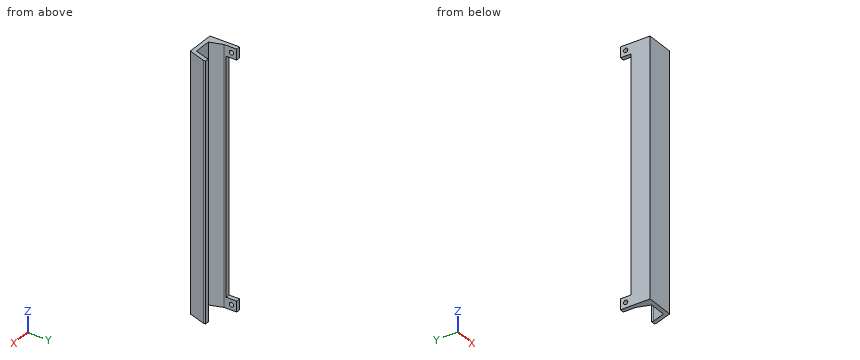
Autodesk Inventor part; units mm, degrees
ref_plane "YZ Plane" through (0, 0, 0) normal (1, 0, 0) x (0, 1, 0)
ref_plane "XZ Plane" through (0, 0, 0) normal (0, 1, 0) x (-1, 0, 0)
ref_plane "XY Plane" through (0, 0, 0) normal (0, 0, 1) x (1, 0, 0)
sketch "Sketch1" plane through (0, 0, 0) normal (0, 0, 1) x (1, 0, 0)
  circle A0 centre (0, 0) radius 7.62
  line L0 (-7.62, 0) -> (-7.62, 1.27)
  line L1 (0, -7.62) -> (-5.08, -7.62)
  line L2 (0, -7.62) -> (5.08, -7.62)
  line L3 (-7.62, 0) -> (-5.08, -7.62)
  line L4 (5.08, -7.62) -> (7.62, 0)
  line L5 (7.62, 0) -> (7.62, 1.27)
  line L6 (-7.62, 1.27) -> (-10.16, 1.27)
  line L7 (-10.16, 1.27) -> (-10.16, 0)
  line L8 (-5.08, -7.62) -> (-6.7733, -10.16)
  line L9 (-6.7733, -10.16) -> (-10.16, 0)
  line L10 (7.62, 1.27) -> (10.16, 1.27)
  line L11 (10.16, 1.27) -> (10.16, 0)
  line L12 (10.16, 0) -> (6.7733, -10.16)
  line L13 (6.7733, -10.16) -> (-6.7733, -10.16)
  line L14 (5.08, -7.62) -> (6.7733, -10.16)
  dimension "d0" = 15.24
  dimension "d1" = 1.27
  dimension "d2" = 5.08
  dimension "d3" = 5.08
  dimension "d4" = 1.27
  dimension "d6" = 2.54
  dimension "d7" = 2.54
  dimension "d8" = 2.54
extrude "Extrusion1" add sketch "Sketch1" along normal blind 152.4 contours L5 L10 L11 L12 L14 L4 A0 | A0 L4 | L3 A0 | A0 L3 L8 L9 L7 L6 L0 | L2 L14 L13 L8 L1
sketch "Sketch2" plane through (-7.62, 1.27, 152.4) normal (1, 0, 0) x (0, 0, -1)
  point P0 (152.4, -1.27)
sketch "Sketch3" plane through (0, 0, 152.4) normal (0, 0, 1) x (1, 0, 0)
  line L0 (-10.16, 1.27) -> (-10.16, 0)
  line L1 (-10.16, 0) -> (-10.16, -10.16)
  line L2 (-6.7733, -10.16) -> (6.7733, -10.16)
  line L3 (-10.16, -10.16) -> (-6.7733, -10.16)
  line L4 (-10.16, 0) -> (-6.7733, -10.16)
  point P0 (0, 0)
extrude "Extrusion2" add sketch "Sketch3" against normal up to surface (152.4 mm away)
sketch "Sketch4" plane through (-7.62, 1.27, 152.4) normal (1, 0, 0) x (0, 0, -1)
  line L0 (152.4, -1.27) -> (152.4, 0)
  line L1 (152.4, 0) -> (146.05, 0)
  line L2 (146.05, 0) -> (146.05, 6.35)
  line L3 (146.05, 6.35) -> (152.4, 6.35)
  line L4 (152.4, 6.35) -> (152.4, 0)
  circle A0 centre (149.225, 3.175) radius 1.27
  line L5 (152.4, 0) -> (0, 0)
  line L6 (76.2, 0) -> (76.2, 6.35)
  line L7 (76.2, 0) -> (82.55, 0) construction
  line L8 (6.35, 0) -> (6.35, 6.35)
  line L9 (6.35, 6.35) -> (0, 6.35)
  line L10 (0, 6.35) -> (0, 0)
  circle A1 centre (3.175, 3.175) radius 1.27
  dimension "d13" = 6.35
  dimension "d14" = 6.35
  dimension "d15" = 2.54
  dimension "d16" = 3.175
  dimension "d17" = 3.175
  dimension "d18" = 6.35
  dimension "d19" = 90
extrude "Extrusion3" add sketch "Sketch4" against normal up to surface (2.54 mm away)
properties part number "StraightTrackv2"
The listing builds one solid part. Answer for the finished solid, in the listing's coordinates (mm). Coordinates: 2 decimals unless noted, no trailing zeros. Write each loop counter-clockwise with the first axis right and the second up, starting at its lowest first coordinate (ties: lowest second). Pieces come first, ordered by that corner, then holes. Notation, with made-up numbers: M 21,34.5 L 39,34.5 A18 cw 39,44.5 Z; hole C 39,-9 d3. An arc over 180 degrees is marked long. Put each result on its own line as item: value. Start each with the question number.
1. A cutting plane is placed at B-B on z = 11. Write down the section's boundary in (x, y).
2. Flat-ended cylindrical pins translate along their axes: P1, Ø6, axis at y = -4, z = 96, coming from the +X side; P2, Ø6, axis at x = -1, z = 42.5, coming from the +Y side; P3, Ø1.3, axis at x = 8.5, z = 73, coming from the +Y side. Find the tip coordinate at first contact, or state that the pin passes through.
3. A cutting plane is placed at C-C on x = 0. Write down the section's boundary in (y, z), then the cut area to 3 significant figures.
4. Consider line 1 (X direction, y = 1, z = 95); line 2 (Z direction, x = -8.75, y = 5); line 3 (Y direction, x = -1, z = 121.5). Determine where each line is inside the solid, lowest interval first. Write a range as from..to.
5. A cutting plane is placed at A-A on y = -3.75. Write down the section's boundary in (x, z).
Resolved:
1. outline: M -10.16,-10.16 L 6.77,-10.16 L 10.16,0 L 10.16,1.27 L 7.62,1.27 L 7.62,0 L 5.08,-7.62 L -5.08,-7.62 L -7.62,0 L -7.62,1.27 L -10.16,1.27 Z
2. P1: stops at x = 9.83
2. P2: stops at y = -7.62
2. P3: stops at y = 1.27
3. outline: M -10.16,0 L -7.62,0 L -7.62,152.4 L -10.16,152.4 Z
3. area: 387 mm2
4. line 1: x = -10.16..-7.62, 7.62..10.16
4. line 2: z = 0..2.03, 4.32..6.35, 146.05..148.08, 150.37..152.4
4. line 3: y = -10.16..-7.62
5. outline: M -10.16,0 L -6.37,0 L -6.37,152.4 L -10.16,152.4 Z; M 6.37,0 L 8.91,0 L 8.91,152.4 L 6.37,152.4 Z
